For this review, take the finished solid that the model builds, in its own axes (mm). Face numbers are marked on the shaded views. A direction names the side the tool comes from. Coordinates: 2 decimals unless noted, no trailing zeros. Loops run counter-clockwise (first coordinate to the right, second up) from the corner with the lowest first, then second, coordinate; pieces in that order, holes last. Notation, with made-up numbers: (58.25, -24) -> (83.25, -24) arc R30 ccw to (83.25, 9) -> close; hole circle Ø4 at (18.5, 84.25). An arc over 180 degrees is marked (long way). Answer in a Markdown table with one row per item.
from build123d import *

# Parameters (mm, degrees)
SKETCH1_R           = 2
SKETCH1_W           = 15.1
SKETCH1_H           = 5.1
BOSS_EXTRUDE1_DEPTH = 5


with BuildPart() as part:
    # Sketch1 → Boss-Extrude1 (new body)
    with BuildSketch(Plane.XY):
        Polygon((-70.2, 20), (-65.2, 20), (-65.2, 0), (-60.1, 0), (-60.1, 15), (-55.1, 15), (-55.1, 0), (-50.1, 0), (-50.1, -20), (-10, -20), (-10, 0), (0, 0), (0, -20), (-5, -20), (-5, -25), (-20.2, -25), (-20.2, -35), (-45.2, -35), (-45.2, -25), (-60.2, -25), (-60.2, -20), (-70.2, -20), align=None)
        with Locations((-54.1, -5)):
            Circle(SKETCH1_R, mode=Mode.SUBTRACT)
        with Locations((-54.1, -15)):
            Circle(SKETCH1_R, mode=Mode.SUBTRACT)
        with Locations((-6, -5)):
            Circle(SKETCH1_R, mode=Mode.SUBTRACT)
        with Locations((-6, -15)):
            Circle(SKETCH1_R, mode=Mode.SUBTRACT)
        with Locations((-32.75, -27.45)):
            Rectangle(SKETCH1_W, SKETCH1_H, mode=Mode.SUBTRACT)
    extrude(amount=BOSS_EXTRUDE1_DEPTH)


solid = part.part
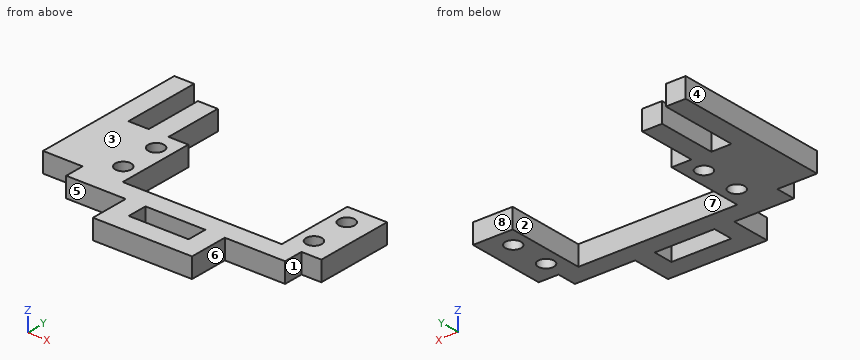
Item 1: Take a section at D-D, the plane x = -37. State the section outline as (y, z) points, and give its area (3 significant figures).
Worked answers:
| item | result |
|---|---|
| outline | (-35, 0) -> (-30, 0) -> (-30, 5) -> (-35, 5) -> close; (-24.9, 0) -> (-20, 0) -> (-20, 5) -> (-24.9, 5) -> close |
| area | 49.5 mm² |
Item 2: Take a section at B-B, the plane z = 1.75. Count the separate pieces of the cut face and the enclosed holes in it, and give its area (3 significant figures).
Worked answers:
| item | result |
|---|---|
| separate pieces | 1 |
| enclosed holes | 5 |
| area | 1,180 mm² |
Item 3: For the marked faces 4, 5, 6, 7 and 8, list the 3-axis set-ups (+Z, -Z, +X, -X, +Y, -Y) from which the entire face can be reached by the end or side of a thin tool; tool diameter is ignored.
Worked answers:
| item | result |
|---|---|
| face 4 | +Z, -Z, -X, +Y, -Y |
| face 5 | +Z, -Z, -X, -Y |
| face 6 | +Z, -Z, +X, -Y |
| face 7 | +Z, -Z, +Y |
| face 8 | +Z, -Z, +X, +Y |
Item 4: Take a section at A-A, the plane x = -54.1. State the section outline as (y, z) points, and give its area (3 significant figures).
Worked answers:
| item | result |
|---|---|
| outline | (-25, 0) -> (-17, 0) -> (-17, 5) -> (-25, 5) -> close; (-13, 0) -> (-7, 0) -> (-7, 5) -> (-13, 5) -> close; (-3, 0) -> (0, 0) -> (0, 5) -> (-3, 5) -> close |
| area | 85.0 mm² |
Item 5: Insertion check: pin 1 (2.5 mm diameter, centred on x = -6, y = -15, fed in from -Z) (3 decimals); pin 2 (2.5 mm diameter, centred on x = -53, z = 3, fed in from +Y); pin 3 (2.5 mm diameter, centred on y = -28, z = 3.5, fed in from -X); pin 4 (2 mm diameter, centred on y = -24, z = 0.5, fed in from +X). Each pin has a flat end and moves straight along its axis. Give the tip position at first contact, or say it passes through.
Worked answers:
| item | result |
|---|---|
| pin 1 | through |
| pin 2 | y = 0 |
| pin 3 | x = -45.2 |
| pin 4 | x = -5 |
Item 6: For L1, parallel to Y at x = -54.1, z = 1.55; L2, parallel to X at y = 2.5, z = 3.05; L3, parallel to Y at x = -31.5, z = 3.05, list the stretches that pass through material, from the lowest coordinate up.
Worked answers:
| item | result |
|---|---|
| L1 | -25 to -17, -13 to -7, -3 to 0 |
| L2 | -70.2 to -65.2, -60.1 to -55.1 |
| L3 | -35 to -30, -24.9 to -20 |
Item 7: Take a section at C-C, the plane y = -5. State the section outline as (x, z) points, and give its area (4 significant figures).
Worked answers:
| item | result |
|---|---|
| outline | (-70.2, 0) -> (-56.1, 0) -> (-56.1, 5) -> (-70.2, 5) -> close; (-52.1, 0) -> (-50.1, 0) -> (-50.1, 5) -> (-52.1, 5) -> close; (-10, 0) -> (-8, 0) -> (-8, 5) -> (-10, 5) -> close; (-4, 0) -> (0, 0) -> (0, 5) -> (-4, 5) -> close |
| area | 110.5 mm² |
Item 8: The part is to be moulded in two halves that separate along X. For the marked faces 1, 2 and 3, say which applies: +X half, -X half, draft (parallel to the pull), parting line (faces both ways), or undercut.
Worked answers:
| item | result |
|---|---|
| face 1 | +X half |
| face 2 | undercut |
| face 3 | draft |
